Could you check a few things on this model? Use its own coordinates, in mm. A direction names the side the tool comes from. Give positions to 0.01 mm unless a question says otherwise; leave off trailing zeros. Write each loop counter-clockwise with the first axis right and the second up, starting at its lowest first coordinate (ties: lowest second). Pieces come first, ordered by that corner, then holes. Notation, with made-up numbers: (-10.75, 70.25) -> (-3.75, 70.25) arc R13 cw to (-3.75, 75.25) -> close; hole circle Ø1 at (-20.5, -18.75). An arc over 180 degrees is marked (long way). Write item = value, one per line. Start each with the question number.
```python
from build123d import *

# Parameters (mm, degrees)
SKETCH2_R            = 6.5
SKETCH2_R_2          = 0.5
SKETCH2_R_3          = 2
BOSS_EXTRUDE2_DEPTH  = 6
SKETCH2_14_R         = 2
BOSS_EXTRUDE9_DEPTH  = 20
BOSS_EXTRUDE5_START  = 6
SKETCH2_7_R          = 8.5
SKETCH2_7_R_2        = 6.5
BOSS_EXTRUDE5_DEPTH  = 15
BOSS_EXTRUDE10_START = 3
SKETCH2_16_R         = 6.5
SKETCH2_16_R_2       = 4
BOSS_EXTRUDE10_DEPTH = 15
RIB20_REACH          = 60.526
SKETCH6_WALL_W       = 131.852983596
SKETCH6_WALL_H       = 10


with BuildPart() as part:
    # Sketch2 → Boss-Extrude2 (new body)
    with BuildSketch(Plane.XY):
        with BuildLine():
            Line((10.269230614, 13.695123544), (24.482427586, 26.279928647))
            ThreePointArc((24.482427586, 26.279928647), (32.678156537, 40.21498183), (17.85326379, 33.766863091))
            Line((17.85326379, 33.766863091), (3.640066818, 21.182057988))
            ThreePointArc((3.640066818, 21.182057988), (-14.86387718, -1.880208276), (10.269230614, 13.695123544))
        make_face()
        with Locations((26.31426226, 34.580192603)):
            Circle(SKETCH2_R, mode=Mode.SUBTRACT)
        with Locations((2.730418762, 13.698326645)):
            Circle(SKETCH2_R_2, mode=Mode.SUBTRACT)
        with Locations((-9.997369792, 2.428748191)):
            Circle(SKETCH2_R_2, mode=Mode.SUBTRACT)
        with Locations((1.006939142, 2.822683307)):
            Circle(SKETCH2_R_2, mode=Mode.SUBTRACT)
        with Locations((-8.273890172, 13.304391529)):
            Circle(SKETCH2_R_2, mode=Mode.SUBTRACT)
        with Locations((-3.633475515, 8.063537418)):
            Circle(SKETCH2_R_3, mode=Mode.SUBTRACT)
    extrude(amount=BOSS_EXTRUDE2_DEPTH)

    # Sketch2<14> → Boss-Extrude9 (add)
    with BuildSketch(Plane.XY):
        with Locations((-3.633475515, 8.063537418)):
            Circle(SKETCH2_14_R)
    extrude(amount=BOSS_EXTRUDE9_DEPTH)

    # Sketch2<7> → Boss-Extrude5 (add)
    with BuildSketch(Plane.XY.offset(BOSS_EXTRUDE5_START)):
        with Locations(Location((26.31426226, 34.580192603, 0), (0, 0, 185.490794513))):
            Circle(SKETCH2_7_R)
        with Locations((26.31426226, 34.580192603)):
            Circle(SKETCH2_7_R_2, mode=Mode.SUBTRACT)
    extrude(amount=BOSS_EXTRUDE5_DEPTH)

    # Sketch2<16> → Boss-Extrude10 (add)
    with BuildSketch(Plane.XY.offset(BOSS_EXTRUDE10_START)):
        with Locations((26.31426226, 34.580192603)):
            Circle(SKETCH2_16_R)
        with Locations((26.31426226, 34.580192603)):
            Circle(SKETCH2_16_R_2, mode=Mode.SUBTRACT)
    extrude(amount=BOSS_EXTRUDE10_DEPTH)

    # Sketch6 wall → Rib20 (add, up to next)
    with BuildSketch(Plane(origin=(16.066946169, 25.506901345, 9.75), x_dir=(-0.606734584094, -0.537221605037, -0.585889146124), z_dir=(-0.438651362827, -0.388395511607, 0.810391207044)), mode=Mode.PRIVATE) as rib20_sk1:
        Rectangle(SKETCH6_WALL_W, SKETCH6_WALL_H)
    rib20_tool1 = extrude(rib20_sk1.sketch, amount=-RIB20_REACH, mode=Mode.PRIVATE) - part.part
    add(rib20_tool1.solids().sort_by_distance((16.066946169, 25.506901345, 9.75))[0])


solid = part.part
```
(1) I'm going to push flat-ended pins straight in: pin 1 (3 mm diameter, centred on y = 30, z = 9, fed in from +X); pin 2 (11.5 mm diameter, centred on x = 26.31, y = 34.58, fed in from -Z); pin 3 (10.5 mm diameter, centred on x = 26.31, y = 34.58, fed in from +Z). Where does each tip first touch, or does it pass through?
(2) Imagine slicing it at A-A (x = 28). Please give me the cut outline in (y, z).
(3) Imagine slicing it at D-D (y = 37.5). Please give me the cut outline in (x, z), then the cut area to 3 significant figures.
(4) We'd pull the mould along X, two halves only. Please class faces 4 (the flat face through (23, 32, 3)), 5 (the flat face through (16.785, 26.049, 10.399)), 6 (the cylindrical face through (-2.71, 6.29, 12.9)): released by +X, released by -X, zero draft, split by the parting line, or undercut.
(5) Imagine slicing it at B-B (z = 9.75). Please give me the cut outline in (x, y), then the cut area to 3 significant figures.
(6) If I drill on line 1 along X through (y, z) = (2.5, 1.5) (3 decimals); line 2 along Z through (x, y) = (-5, 9); line 3 along Z through (x, y) = (-7, -1.5), over which ranges is the centre line in solid material (lowest first)? Write a range as from..to.
(7) On a 3-axis mill with a long thin cutter (end or side, diameter ignored), from which of +Z, -Z, +X, -X, +Y, -Y can I reach the whole of each face in a straight line? I mean faces 1 (the flat face through (-4, 8, 20)), 2 (the flat face through (23, 32, 18)), 3 (the cylindrical face through (32.514, 36.533, 1.479)). Say none if no direction works.
(8) Imagine slicing it at C-C (z = 1.75). Please give me the cut outline in (x, y), then the cut area to 3 significant figures.
Answers below:
q1.pin_1 = 34.24
q1.pin_2 = 3
q1.pin_3 = 18
q2.outline = (26.25, 0) -> (28.3, 0) -> (28.3, 3) -> (30.95, 3) -> (30.95, 18) -> (28.3, 18) -> (28.3, 21) -> (26.25, 21) -> close; (38.21, 3) -> (40.86, 3) -> (40.86, 0) -> (42.91, 0) -> (42.91, 21) -> (40.86, 21) -> (40.86, 18) -> (38.21, 18) -> close
q3.outline = (18.33, 0) -> (20.51, 0) -> (20.51, 3) -> (23.58, 3) -> (23.58, 18) -> (20.51, 18) -> (20.51, 21) -> (18.33, 21) -> close; (29.05, 3) -> (32.12, 3) -> (32.12, 0) -> (34.3, 0) -> (34.3, 21) -> (32.12, 21) -> (32.12, 18) -> (29.05, 18) -> close
q3.area = 184 mm^2
q4.face_4 = undercut
q4.face_5 = released by -X
q4.face_6 = split by the parting line
q5.outline = circle Ø4 at (-3.63, 8.06); (12.75, 29.25) -> (19.38, 21.76) -> (24.48, 26.28) arc R8.5 ccw (long way) to (17.85, 33.77) -> close; hole circle Ø8 at (26.31, 34.58)
q5.area = 246 mm^2
q6.line_1 = -17.564..-10.492, -9.502..0.625, 1.389..10.297
q6.line_2 = 0..20
q6.line_3 = 0..6
q7.face_1 = +Z, +X, -X, +Y, -Y
q7.face_2 = +Z
q7.face_3 = -Z
q8.outline = (3.64, 21.18) arc R15 ccw (long way) to (10.27, 13.7) -> (24.48, 26.28) arc R8.5 ccw (long way) to (17.85, 33.77) -> close; hole circle Ø1 at (-10, 2.43); hole circle Ø1 at (-8.27, 13.3); hole circle Ø1 at (1.01, 2.82); hole circle Ø1 at (2.73, 13.7); hole circle Ø13 at (26.31, 34.58)
q8.area = 971 mm^2
